Here's the drawing with two shaded views (mm, measured from the low corner). I have some questions. Round coordinates to 2 decimals unless told otherwise and drop trailing zeros. Order: outer loops, then holes, each group sorted by start corner. A loop starts at its lowest first (then second) coordinate and runs counter-clockwise, first axis right, second up. Notation, with made-up numbers: (61, 28) -> (70, 28) arc R16 cw to (70, 57) -> close; hole circle Ø8 at (2.5, 52.25). An arc over 180 degrees is marked (long way). Use a Markdown table: item, result. Add a question column.
Q1. I need wall thicknesses on line 1 along X through (y, z) = (19.05, 2.5); line 2 along X through (y, z) = (15, 4.05) (1 decimal); line 3 along Y through (x, z) = (228, 1.75). Which ranges of each line are inside material? Lowest first, please. Write a range as [from, to].
Q2. If we section it at A-A on y = 19.05: List the corners of the cut face in (x, z) for me.
Q3. If we section it at B-B on z = 3.95: Give the number of separate pieces and of enclosed holes in the cut face, plus the area to 3 significant figures.
Q4. I'm going to push a flat-ended pin straight in: pin 1 Ø5.5 at (x, y) = (229.28, 19.05) entering from -Z. Where does the tip first touch, or does it pass through?
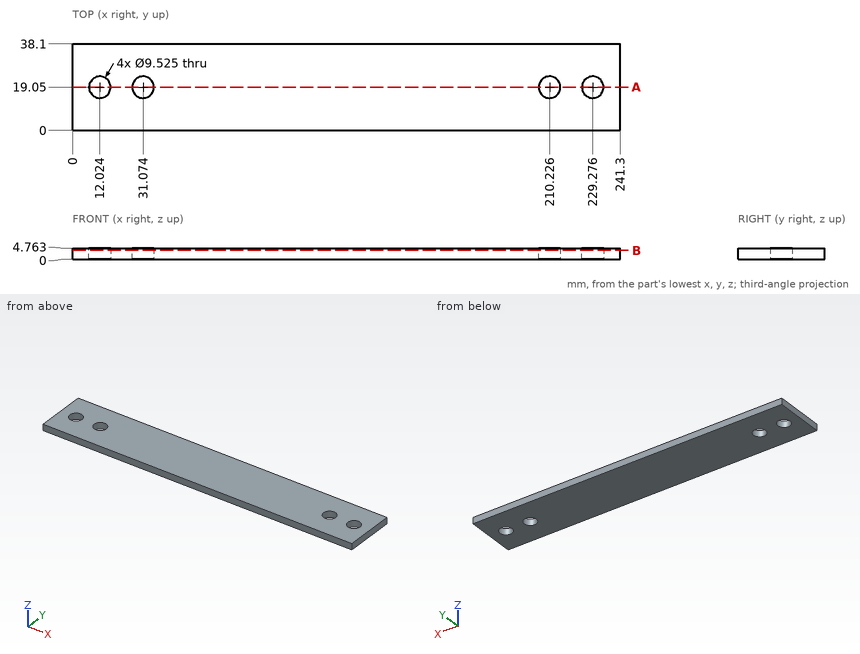
Answer below:
| question | item | result |
|---|---|---|
| 1 | line 1 | [0, 7.26], [16.79, 26.31], [35.84, 205.46], [214.99, 224.51], [234.04, 241.3] |
| 1 | line 2 | [0, 9.5], [14.5, 28.6], [33.6, 207.7], [212.7, 226.8], [231.8, 241.3] |
| 1 | line 3 | [0, 14.46], [23.64, 38.1] |
| 2 | outline | (0, 0) -> (7.26, 0) -> (7.26, 4.76) -> (0, 4.76) -> close; (16.79, 0) -> (26.31, 0) -> (26.31, 4.76) -> (16.79, 4.76) -> close; (35.84, 0) -> (205.46, 0) -> (205.46, 4.76) -> (35.84, 4.76) -> close; (214.99, 0) -> (224.51, 0) -> (224.51, 4.76) -> (214.99, 4.76) -> close; (234.04, 0) -> (241.3, 0) -> (241.3, 4.76) -> (234.04, 4.76) -> close |
| 3 | separate pieces | 1 |
| 3 | enclosed holes | 4 |
| 3 | area | 8,910 mm² |
| 4 | pin 1 | through |
